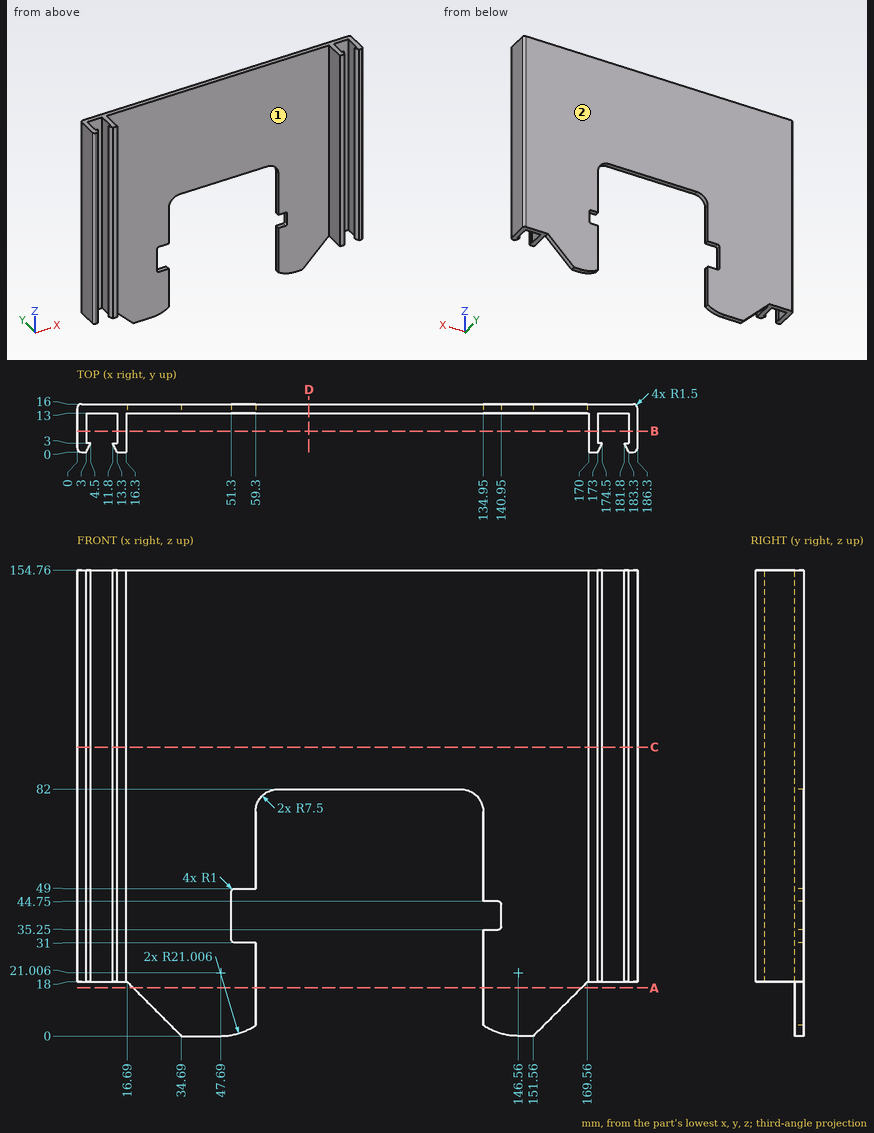
Here's the drawing with two shaded views (mm, measured from the low corner). I have some questions. Coordinates: 2 decimals unless noted, no trailing zeros. Write each loop counter-clockwise with the first axis right and the second up, starting at its lowest first coordinate (ties: lowest second). Pieces come first, ordered by that corner, then holes. Notation, with made-up numbers: M -39.5,-10 L 10.5,-10 A18 ccw 10.5,24 Z; hole C 2.25,64 d3. An arc over 180 degrees is marked long. Answer as CSV lines item,"result".
Item 1: I'm going to push flat-ended pins straight in: P1, Ø2, axis at x = 154.5, z = 95.5, coming from the -Y side; P2, Ø0.9, axis at x = 98.5, y = 14.5, coming from the -Z side; P3, Ø8, axis at x = 6, y = 9.5, coming from the -Z side. Where does each tip first touch, or does it pass through?
Geometry results:
P1,"stops at y = 13"
P2,"stops at z = 82"
P3,"stops at z = 18"
Item 2: Imagine slicing it at D-D on x = 77. List the corners of the cut face in (y, z) for me.
Geometry results:
outline,"M 13,82 L 16,82 L 16,154.76 L 13,154.76 Z"
Item 3: We'd pull the mould along X, two halves only. Please class the marked faces 1 and 2: +X half, -X half, draft (parallel to the pull), parting line (faces both ways), or undercut.
Geometry results:
face 1,"undercut"
face 2,"draft"
Item 4: Imagine slicing it at B-B on y = 7. List the corners of the cut face in (x, z) for me.
Geometry results:
outline,"M 0,18 L 3,18 L 3,154.76 L 0,154.76 Z; M 13.3,18 L 16.3,18 L 16.3,154.76 L 13.3,154.76 Z; M 170,18 L 173,18 L 173,154.76 L 170,154.76 Z; M 183.3,18 L 186.3,18 L 186.3,154.76 L 183.3,154.76 Z"
Item 5: Imagine slicing it at C-C on z = 96. List the corners of the cut face in (x, y) for me.
Geometry results:
outline,"M 0,1.5 A1.5 ccw 1.5,0 L 3,0 L 4.5,3 L 3,3 L 3,13 L 13.3,13 L 13.3,3 L 11.8,3 L 13.3,0 L 16.3,0 L 16.3,13 L 170,13 L 170,0 L 173,0 L 174.5,3 L 173,3 L 173,13 L 183.3,13 L 183.3,3 L 181.8,3 L 183.3,0 L 184.8,0 A1.5 ccw 186.3,1.5 L 186.3,14.5 A1.5 ccw 184.8,16 L 1.5,16 A1.5 ccw 0,14.5 Z"
Item 6: Imagine slicing it at A-A on z = 16. List the corners of the cut face in (x, y) for me, plus the area to 3 significant figures.
Geometry results:
outline,"M 18.69,13 L 59.3,13 L 59.3,16 L 18.69,16 Z; M 134.95,13 L 167.56,13 L 167.56,16 L 134.95,16 Z"
area,"220 mm2"
Item 7: Please list where these lines run through material, in increasing order: line 1 along X through (y, z) = (4.25, 45.5); line 2 along X through (y, z) = (2, 52.5); line 3 along Z through (x, y) = (94.5, 14.75).
Geometry results:
line 1,"x = 0 to 3, 13.3 to 16.3, 170 to 173, 183.3 to 186.3"
line 2,"x = 0 to 4, 12.3 to 16.3, 170 to 174, 182.3 to 186.3"
line 3,"z = 82 to 154.76"
